from build123d import *

# Parameters (mm, degrees)
ESBO_O2_W                     = 30.045415171
ESBO_O2_H                     = 30
RESSALTO_EXTRUS_O1_DEPTH      = 255
ESBO_O4_W                     = 100
ESBO_O4_H                     = 35
RESSALTO_EXTRUS_O2_DEPTH      = 0.001
RESSALTO_EXTRUS_O2_DEPTH_BACK = 3
FILETE1_R                     = 5
FILETE2_R                     = 10


with BuildPart() as part:
    # Esboço2 → Ressalto-extrusão1 (new body, symmetric)
    with BuildSketch(Plane.XY):
        with Locations((-95.635568537, 15)):
            Rectangle(ESBO_O2_W, ESBO_O2_H)
    extrude(amount=RESSALTO_EXTRUS_O1_DEPTH, both=True)

    # Esboço4 → Ressalto-extrusão2 (add, two sides)
    with BuildSketch(Plane.XY.offset(40)) as ressalto_extrus_o2_sk:
        with Locations((-60.658276122, 47.5)):
            Rectangle(ESBO_O4_W, ESBO_O4_H)
    extrude(amount=RESSALTO_EXTRUS_O2_DEPTH)
    extrude(ressalto_extrus_o2_sk.sketch, amount=-RESSALTO_EXTRUS_O2_DEPTH_BACK)

    # Filete1
    filete1_edges = [part.edges().sort_by_distance(p)[0] for p in [
        (-95.635568536, 30, 37),
        (-95.635568536, 30, 40.001),
    ]]
    fillet(filete1_edges, radius=FILETE1_R)

    # Filete2
    filete2_edges = [part.edges().sort_by_distance(p)[0] for p in [
        (-10.658276122, 65, 38.5005),
        (-10.658276122, 30, 38.5005),
    ]]
    fillet(filete2_edges, radius=FILETE2_R)


solid = part.part
Verification items for the finished model (mm, model axes). A direction names the side the tool comes from. Give positions to 0.01 mm unless a question says otherwise; leave off trailing zeros. Loops run counter-clockwise (first coordinate to the right, second up) from the corner with the lowest first, then second, coordinate; pieces in that order, holes last.
1. Cross-section at C-C on z = -184. Record the cut outline in (x, y).
Derived:
outline: (-110.66, 0) - (-80.61, 0) - (-80.61, 30) - (-110.66, 30) - close
2. Tool access check on faces 1 (the flat face through (-96, 30, 151)), 2 (the flat face through (-96, 30, -109)), 3 (the flat face through (-96, 15, 255)). Record the directions out of +Z, -Z, +X, -X, +Y, -Y that give a thin tool (end or side, any length) a straight path to the whole face; none if there is none.
Derived:
face 1: +Z, +X, -X, +Y
face 2: -Z, +X, -X, +Y
face 3: +Z, +X, -X, +Y, -Y
3. Cross-section at B-B on y = 12.5. Record the cut outline in (x, z), and give its area (3 significant figures).
Derived:
outline: (-110.66, -255) - (-80.61, -255) - (-80.61, 255) - (-110.66, 255) - close
area: 15,300 mm2
4. Cross-section at A-A on x = -90. Record the cut outline in (y, z).
Derived:
outline: (0, -255) - (30, -255) - (30, 32) arc R5 cw to (35, 37) - (65, 37) - (65, 40) - (35, 40) arc R5 cw to (30, 45) - (30, 255) - (0, 255) - close
5. Go/stop test with flat-tipped pins: P1, Ø5, axis at x = -30.5, y = 51, coming from the -Z side; P2, Ø5, axis at x = -82.5, y = 45.5, coming from the +Z side; P3, Ø24, axis at x = -89, z = 123, coming from the +Y side. Record where each tip stops, or that it passes through.
Derived:
P1: stops at z = 37
P2: stops at z = 40
P3: stops at y = 30
6. Material ranges on probe 1 along Y at (x, z) = (-84, -7); probe 2 along Z at (x, y) = (-17.5, 47); probe 3 along X at (y, z) = (3, 29.5), recorded low to high.
Derived:
probe 1: y = 0 to 30
probe 2: z = 37 to 40
probe 3: x = -110.66 to -80.61
